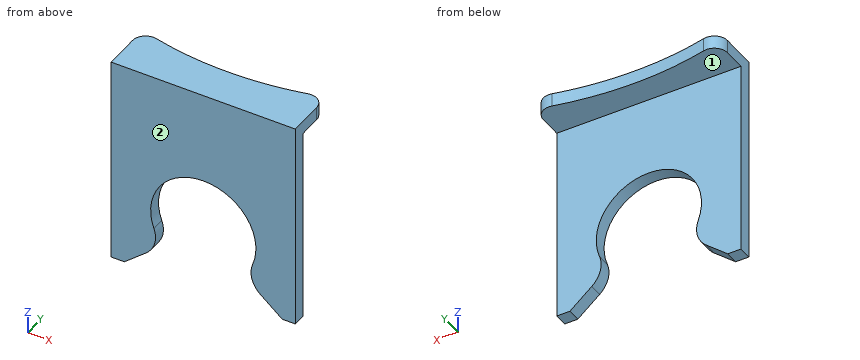
from build123d import *

# Parameters (mm, degrees)
EXTRUDE1_DEPTH = 1
EXTRUDE2_DEPTH = 1
FILLET1_R      = 1


with BuildPart() as part:
    # Sketch1 → Extrude1 (new body)
    with BuildSketch(Plane(origin=(0, 0, 0), x_dir=(1, 0, 0), z_dir=(0, 1, 0))):
        with BuildLine():
            Line((-7, 8), (-6, 8))
            Line((-6, 8), (-4.34571581, 6.621429842))
            ThreePointArc((-4.34571581, 6.621429842), (-3.693602337, 5.600266108), (-3.750723073, 4.389991522))
            ThreePointArc((-3.750723073, 4.389991522), (0, -1), (3.750723073, 4.389991522))
            ThreePointArc((3.750723073, 4.389991522), (3.693602337, 5.600266108), (4.34571581, 6.621429842))
            Line((4.34571581, 6.621429842), (6, 8))
            Line((6, 8), (7, 8))
            Line((7, 8), (7, -8))
            Line((7, -8), (-7, -8))
            Line((-7, -8), (-7, 8))
        make_face()
    extrude(amount=EXTRUDE1_DEPTH)

    # Sketch2 → Extrude2 (add)
    with BuildSketch(Plane.XY.offset(8)):
        with BuildLine():
            Line((-7, 0), (7, 0))
            Line((7, 0), (7, 4))
            ThreePointArc((7, 4), (0, 3), (-7, 4))
            Line((-7, 4), (-7, 0))
        make_face()
    extrude(amount=-EXTRUDE2_DEPTH)

    # Fillet1
    fillet1_edges = [part.edges().sort_by_distance(p)[0] for p in [
        (-7, 4, 7.5),
        (7, 4, 7.5),
    ]]
    fillet(fillet1_edges, radius=FILLET1_R)


solid = part.part
Verification items for the finished model (mm, model axes). Face numbers are marked on the shaded views. A direction names the side the tool comes from. Coordinates: 2 decimals unless noted, no trailing zeros. Write each loop counter-clockwise with the first axis right and the second up, starting at its lowest first coordinate (ties: lowest second). Pieces come first, ordered by that corner, then holes. Notation, with made-up numbers: (29.25, -31.5) -> (62.25, -31.5) arc R25 cw to (62.25, 6.5) -> close; hole circle Ø3 at (13, -22). An arc over 180 degrees is marked (long way). One line per item, written item: value. Start each with the question number.
Q1. Cross-section at B-B on x = 0. Enter the section's corners in (y, z).
Q2. Access from +Z, -Z, +X, -X, +Y, -Y to the whole of each face (thin tool, end or side, straight path). Record for the marked faces 1 and 2.
Q3. Cross-section at D-D on y = 1.45. Enter the section's corners in (x, z), and give its area (3 significant figures).
Q4. Go/stop test with flat-tipped pins: P1, Ø1, axis at x = 1, y = 1, coming from the -Z side; P2, Ø4, axis at x = 1, z = -2, coming from the +Y side; P3, Ø6, axis at x = -5, z = -1.5, coming from the +Y side; P4, Ø0.8, axis at x = 0.5, y = 2, coming from the -Z side. Record where each tip stops, or that it passes through.
Q5. Thickness scan on L1, parallel to X at y = 0.55, z = -3; L2, parallel to Z at x = -1.25, y = 3; L3, parallel to Y at x = -2, z = 5.75. Record the ranges inside material, lowest first. Write a range as from..to.
Q6. Cross-section at C-C on z = -7. Enter the section's corners in (x, y), and give its area (3 significant figures).
Q7. Cross-section at A-A on z = -3. Enter the section's corners in (x, y).
Checked values:
1. outline: (0, 1) -> (1, 1) -> (1, 7) -> (3, 7) -> (3, 8) -> (0, 8) -> close
2. face 1: -Z, +X, -X, +Y
2. face 2: +Z, -Z, +X, -X, -Y
3. outline: (-7, 7) -> (7, 7) -> (7, 8) -> (-7, 8) -> close
3. area: 14.0 mm²
4. P1: stops at z = 0.71
4. P2: passes through
4. P3: stops at y = 1
4. P4: stops at z = 7
5. L1: x = -7..-4, 4..7
5. L2: z = 7..8
5. L3: y = 0..1
6. outline: (-7, 0) -> (-4.8, 0) -> (-4.8, 1) -> (-7, 1) -> close; (4.8, 0) -> (7, 0) -> (7, 1) -> (4.8, 1) -> close
6. area: 4.40 mm²
7. outline: (-7, 0) -> (-4, 0) -> (-4, 1) -> (-7, 1) -> close; (4, 0) -> (7, 0) -> (7, 1) -> (4, 1) -> close
